Job drawing, mm, ordinate dimensions from the low corner. One solid piece. Round coordinates to 2 decimals unless told otherwise and drop trailing zeros. Write each loop counter-clockwise with the first axis right and the second up, starting at its lowest first coordinate (ties: lowest second). Pieces come first, ordered by that corner, then holes. Notation, with made-up numbers: (9, 63) -> (60, 63) arc R21 cw to (60, 74) -> close; hole circle Ø5 at (86, 17). An arc over 180 degrees is marked (long way). Use CSV: the item, a comma, the result in double quotes. Start each with the question number.
(1) Saw through at B-B (y = 35). Give the cut face in (x, z) (1 decimal), plus the area to 3 significant figures.
(2) Two-plate mould, pull along X, no slides. Class the marked faces 1, 2, 3 and 4: released by +X, released by -X, zero draft, split by the parting line, or undercut.
(3) Drop flat-ended pins along their axis: pin 1 (4 mm diameter, centred on x = 13.88, y = 5.88, fed in from +Z) (3 decimals); pin 2 (1.6 mm diameter, centred on y = 34.5, z = 1.5, fed in from +X); pin 3 (0.8 mm diameter, centred on x = 11.5, z = 1, fed in from -Y); pin 4 (1 mm diameter, centred on y = 34, z = 1, fed in from -X). Give the stop position or say it passes through.
(4) Saw through at C-C (x = 24.75). Give the cut face in (y, z) (1 decimal).
(5) Probe line 1 (Y direction, x = 14, z = 0.6) (1 decimal); line 2 (X direction, y = 7, z = 1.5) (1 decimal); line 3 (Y direction, x = 16.75, z = 1) (1 decimal). List the from-to ranges inside material, lowest first. Write a range as [from, to].
(6) Saw through at A-A (z = 1.65). Give the cut face in (x, y).
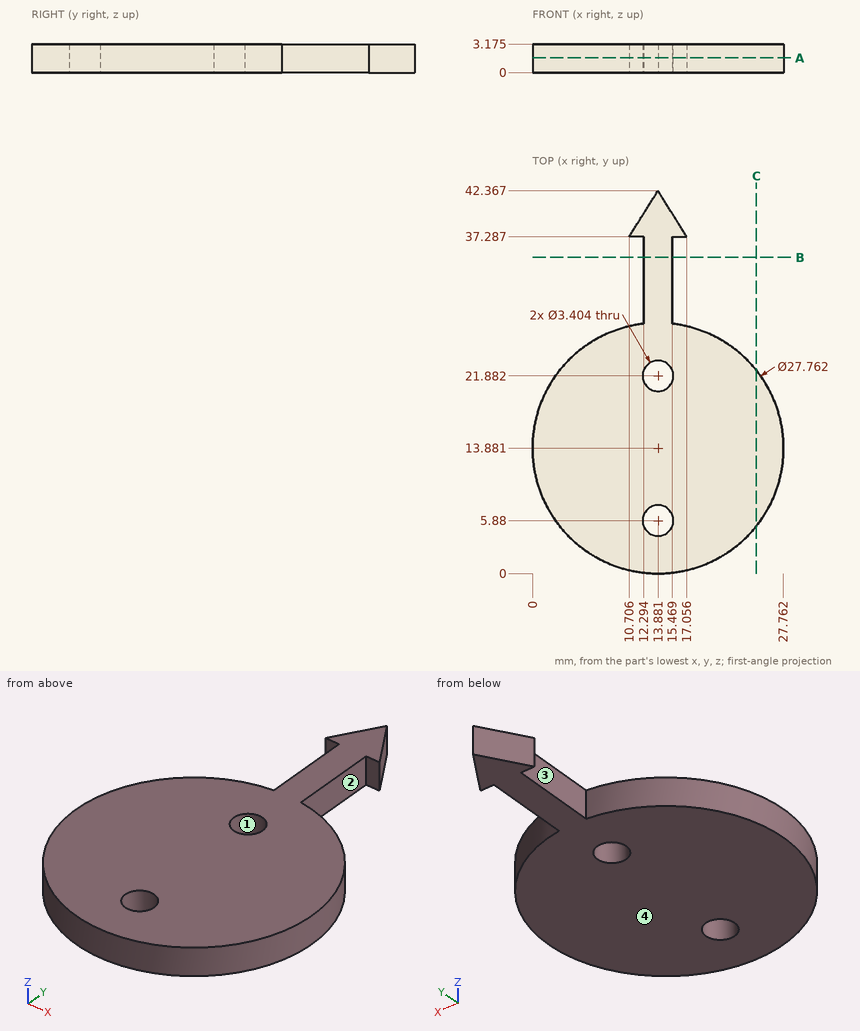
Answers:
1,outline,"(12.3, 0) -> (15.5, 0) -> (15.5, 3.2) -> (12.3, 3.2) -> close"
1,area,"10.1 mm²"
2,face 1,"undercut"
2,face 2,"released by +X"
2,face 3,"released by -X"
2,face 4,"zero draft"
3,pin 1,"stops at z = 3.175"
3,pin 2,"stops at x = 15.47"
3,pin 3,"stops at y = 0.14"
3,pin 4,"stops at x = 12.29"
4,outline,"(5.2, 0) -> (22.5, 0) -> (22.5, 3.2) -> (5.2, 3.2) -> close"
5,line 1,"y = [0, 4.2], [7.6, 20.2], [23.6, 42.2]"
5,line 2,"x = [1.8, 12.6], [15.2, 25.9]"
5,line 3,"y = [0.3, 27.5], [37.3, 37.8]"
6,outline,"(10.71, 37.29) -> (12.29, 37.29) -> (12.29, 27.67) arc R13.88 ccw (long way) to (15.47, 27.67) -> (15.47, 37.29) -> (17.06, 37.29) -> (13.88, 42.37) -> close; hole circle Ø3.4 at (13.88, 5.88); hole circle Ø3.4 at (13.88, 21.88)"
